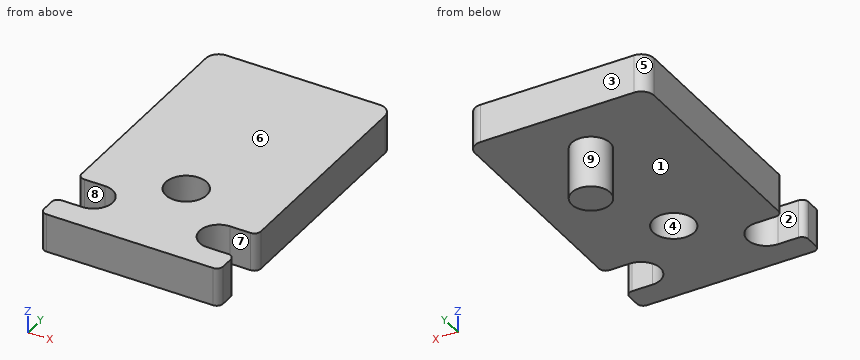
from build123d import *

# Parameters (mm, degrees)
CROQUIS1_R              = 1.6
SALIENTE_EXTRUIR1_DEPTH = 1.5
REDONDEO1_R             = 1
REDONDEO2_R             = 0.5
CROQUIS2_R              = 1.5
SALIENTE_EXTRUIR2_DEPTH = 4


with BuildPart() as part:
    # Croquis1 → Saliente-Extruir1 (new, symmetric)
    with BuildSketch(Plane.XY):
        with BuildLine():
            Line((3, 11.5), (7, 11.5))
            Line((7, 11.5), (7, -6.5))
            Line((7, -6.5), (4.9, -6.5))
            ThreePointArc((4.9, -6.5), (3.4, -8), (4.9, -9.5))
            Line((4.9, -9.5), (7, -9.5))
            Line((7, -9.5), (7, -11.5))
            Line((7, -11.5), (-7, -11.5))
            Line((-7, -11.5), (-7, -9.5))
            Line((-7, -9.5), (-4.9, -9.5))
            ThreePointArc((-4.9, -9.5), (-3.4, -8), (-4.9, -6.5))
            Line((-4.9, -6.5), (-7, -6.5))
            Line((-7, -6.5), (-7, 11.5))
            Line((-7, 11.5), (-3, 11.5))
            Line((-3, 11.5), (3, 11.5))
        make_face()
        with Locations((0, -4)):
            Circle(CROQUIS1_R, mode=Mode.SUBTRACT)
    extrude(amount=SALIENTE_EXTRUIR1_DEPTH, both=True)

    # Redondeo1
    redondeo1_edges = [part.edges().sort_by_distance(p)[0] for p in [
        (-7, 11.5, 0),
        (7, 11.5, 0),
    ]]
    fillet(redondeo1_edges, radius=REDONDEO1_R)

    # Redondeo2
    redondeo2_edges = [part.edges().sort_by_distance(p)[0] for p in [
        (7, -11.5, 0),
        (-7, -11.5, 0),
        (-7, -9.5, 0),
        (-7, -6.5, 0),
        (7, -6.5, 0),
        (7, -9.5, 0),
    ]]
    fillet(redondeo2_edges, radius=REDONDEO2_R)

    # Croquis2 → Saliente-Extruir2 (add)
    with BuildSketch(Plane(origin=(0, 0, -1.5), x_dir=(-1, 0, 0), z_dir=(0, 0, -1))):
        with Locations(Location((0, 7, 0), (0, 0, 180))):
            Circle(CROQUIS2_R)
    extrude(amount=SALIENTE_EXTRUIR2_DEPTH)


solid = part.part
Work out the finished part from the listing and answer in its coordinate system (mm). Face numbers are marked on the shaded views. A direction names the side the tool comes from. Give positions to 0.01 mm unless a question says otherwise; leave off trailing zeros. Write each loop counter-clockwise with the first axis right and the second up, starting at its lowest first coordinate (ties: lowest second). Pieces come first, ordered by that corner, then holes.
Q1. The part is cut by section B-B on y = -4. Give the vertices of the cut face in (x, z).
Answer:
outline: (-7, -1.5) - (-1.6, -1.5) - (-1.6, 1.5) - (-7, 1.5) - close; (1.6, -1.5) - (7, -1.5) - (7, 1.5) - (1.6, 1.5) - close
Q2. The part is cut by section C-C on z = -0.5. Give the vertices of the cut face in (x, y).
Answer:
outline: (-7, -11) arc R0.5 ccw to (-6.5, -11.5) - (6.5, -11.5) arc R0.5 ccw to (7, -11) - (7, -10) arc R0.5 ccw to (6.5, -9.5) - (4.9, -9.5) arc R1.5 cw to (4.9, -6.5) - (6.5, -6.5) arc R0.5 ccw to (7, -6) - (7, 10.5) arc R1 ccw to (6, 11.5) - (-6, 11.5) arc R1 ccw to (-7, 10.5) - (-7, -6) arc R0.5 ccw to (-6.5, -6.5) - (-4.9, -6.5) arc R1.5 cw to (-4.9, -9.5) - (-6.5, -9.5) arc R0.5 ccw to (-7, -10) - close; hole circle Ø3.2 at (0, -4)
Q3. The part is cut by section D-D on y = 7. Give the vertices of the cut face in (x, z).
Answer:
outline: (-7, -1.5) - (-1.5, -1.5) - (-1.5, -5.5) - (1.5, -5.5) - (1.5, -1.5) - (7, -1.5) - (7, 1.5) - (-7, 1.5) - close
Q4. The part is cut by section A-A on x = 0. Give the vertices of the cut face in (y, z), and give its area (3 significant figures).
Answer:
outline: (-11.5, -1.5) - (-5.6, -1.5) - (-5.6, 1.5) - (-11.5, 1.5) - close; (-2.4, -1.5) - (5.5, -1.5) - (5.5, -5.5) - (8.5, -5.5) - (8.5, -1.5) - (11.5, -1.5) - (11.5, 1.5) - (-2.4, 1.5) - close
area: 71.4 mm2
Q5. For a pull along Y with two mould halves and no side action, classify the marked faces 1, 2, 3 and 4 as released by +Y, released by -Y, zero draft, split by the parting line, or undercut.
Answer:
face 1: zero draft
face 2: undercut
face 3: released by +Y
face 4: undercut
Q6. A tool of negligible diameter and unlimited length cuts with its end or side. For the marked faces 5, 6, 7, 8 and 9, from which of +Z, -Z, +X, -X, +Y, -Y can it reach the whole face along a straight path? Write none if from no direction.
Answer:
face 5: +Z, -Z, -X, +Y
face 6: +Z, +X, -X, +Y, -Y
face 7: +Z, -Z, +X
face 8: +Z, -Z, -X
face 9: -Z
Q7. Given pin 1 (3 mm diameter, centred on x = 4, y = -6, fed in from -Z), flat-ended and moving along its own axis, determine where the tip first touches the part or whether it passes through.
Answer:
pin 1: stops at z = -1.5
Q8. Straight lines are drawn through the part: L1, parallel to Y at x = 0, z = 0.2; L2, parallel to Z at x = 4.75, y = 3.75; L3, parallel to Y at x = -6, z = 0.25. For each, find the intervals that lie inside material, in ascending order.
Answer:
L1: y = -11.5 to -5.6, -2.4 to 11.5
L2: z = -1.5 to 1.5
L3: y = -11.5 to -9.5, -6.5 to 11.5
